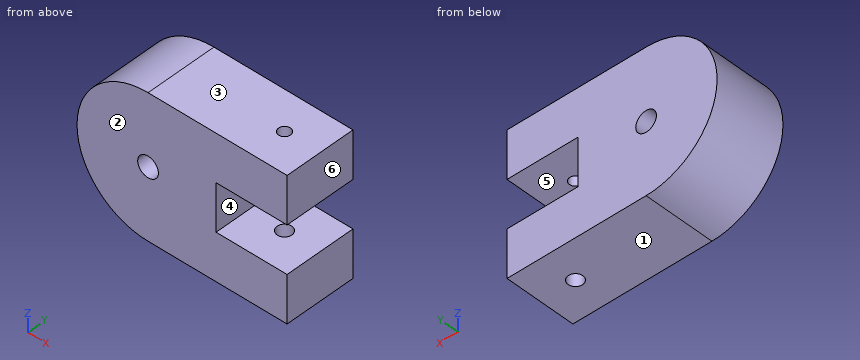
```python
from build123d import *

# Parameters (mm, degrees)
F0_R     = 11.1125
F1_DEPTH = 76.2
F3_R     = 7.9375
F4_DEPTH = 50.8
F2_R     = 6.35
F5_DEPTH = 50.8


with BuildPart() as f1:
    # F0 (on Front) → F1 (new body)
    with BuildSketch(Plane.XZ):
        with BuildLine():
            ThreePointArc((0, 152.4), (-76.2, 76.2), (0, 0))
            Line((0, 0), (149.225, 0))
            Line((149.225, 0), (149.225, 50.8))
            Line((149.225, 50.8), (73.025, 50.8))
            Line((73.025, 50.8), (73.025, 101.6))
            Line((73.025, 101.6), (149.225, 101.6))
            Line((149.225, 101.6), (149.225, 152.4))
            Line((149.225, 152.4), (0, 152.4))
        make_face()
        with Locations((0, 76.2)):
            Circle(F0_R, mode=Mode.SUBTRACT)
    extrude(amount=F1_DEPTH)

    # F3 (on face) → F4 (cut)
    with BuildSketch(Plane(origin=(0, 0, 0), x_dir=(1, 0, 0), z_dir=(0, 0, -1))):
        with Locations((111.125, 38.1)):
            Circle(F3_R)
    extrude(amount=-F4_DEPTH, mode=Mode.SUBTRACT)

    # F2 (on face) → F5 (cut)
    with BuildSketch(Plane.XY.offset(152.4)):
        with Locations((111.125, -38.1)):
            Circle(F2_R)
    extrude(amount=-F5_DEPTH, mode=Mode.SUBTRACT)


solid = f1.part
```
The listing builds one solid part. Answer for the finished solid, in the listing's coordinates (mm). Face numbers are marked on the shaded views. A direction names the side the tool comes from. Give positions to 0.01 mm unless a question says otherwise; leave off trailing zeros. Order: outer loops, then holes, each group sorted by start corner. A loop starts at its lowest first (then second) coordinate and runs counter-clockwise, first axis right, second up. Notation, with made-up numbers: (-16.5, 48.25) -> (7.5, 48.25) arc R15 cw to (7.5, 62.25) -> close; hole circle Ø8 at (17.25, 28). An arc over 180 degrees is marked (long way). Answer as CSV lines item,"result". Start each with the question number.
Q1. Given pin 1 (8 mm diameter, centred on y = -59, z = 77.5, fed in from +X) (3 decimals); pin 2 (6 mm diameter, centred on x = -28, y = -65, fed in from +Z); pin 3 (18 mm diameter, centred on x = 0, z = 76.2, fed in from -Y); pin 4 (6 mm diameter, centred on y = -21, z = 109, fed in from -X), each flat-ended and moving along its own axis, determine where each tip first touches the part or whether it passes through.
Q2. Determine the mould class of the marked faces 1, 2, 3 and 4 for opening direction Z: pulls with the +Z half, pulls with the -Z half, needs draft (parallel to the pull), parting line crosses it, or undercut.
Q3. Which of the six approach directions +Z, -Z, +X, -X, +Y, -Y give full straight-line access (tool end or side, diameter ignored) to the marked faces 5 and 6?
Q4. A cutting plane is placed at A-A (y = -38.1). Determine the outline of the cut face in (x, z) (1 decimal).
Q5. A cutting plane is placed at C-C (z = 76.2). Determine the outline of the cut face in (x, y) (1 decimal), then the cut area to 3 significant figures.
Q6. A cutting plane is placed at B-B (x = 132.5). Determine the outline of the cut face in (y, z), then the cut area to 3 significant figures.
Q7. Find the intervals of material crossed by L1, parallel to Z at x = 0, y = -49; L2, parallel to Z at x = 76, y = -26.5; L3, parallel to X at y = -47, z = 76 (3 decimals), in increasing order.
Q8. A cutting plane is placed at D-D (y = -56.5). Determine the outline of the cut face in (x, z) (1 decimal).
Results found:
1,pin 1,"x = 73.025"
1,pin 2,"z = 148.18"
1,pin 3,"through"
1,pin 4,"x = -70.13"
2,face 1,"pulls with the -Z half"
2,face 2,"needs draft"
2,face 3,"pulls with the +Z half"
2,face 4,"undercut"
3,face 5,"+X, +Y, -Y"
3,face 6,"+Z, -Z, +X, +Y, -Y"
4,outline,"(0, 0) -> (103.2, 0) -> (103.2, 50.8) -> (73, 50.8) -> (73, 101.6) -> (104.8, 101.6) -> (104.8, 152.4) -> (0, 152.4) arc R76.2 ccw to start; (117.5, 101.6) -> (149.2, 101.6) -> (149.2, 152.4) -> (117.5, 152.4) -> close; (119.1, 0) -> (149.2, 0) -> (149.2, 50.8) -> (119.1, 50.8) -> close; hole circle Ø22.2 at (0, 76.2)"
5,outline,"(-76.2, -76.2) -> (-11.1, -76.2) -> (-11.1, 0) -> (-76.2, 0) -> close; (11.1, -76.2) -> (73, -76.2) -> (73, 0) -> (11.1, 0) -> close"
5,area,"9,680 mm2"
6,outline,"(-76.2, 0) -> (0, 0) -> (0, 50.8) -> (-76.2, 50.8) -> close; (-76.2, 101.6) -> (0, 101.6) -> (0, 152.4) -> (-76.2, 152.4) -> close"
6,area,"7,740 mm2"
7,L1,"0 to 65.09, 87.31 to 152.4"
7,L2,"0 to 50.8, 101.6 to 152.4"
7,L3,"-76.2 to -11.111, 11.111 to 73.025"
8,outline,"(0, 0) -> (149.2, 0) -> (149.2, 50.8) -> (73, 50.8) -> (73, 101.6) -> (149.2, 101.6) -> (149.2, 152.4) -> (0, 152.4) arc R76.2 ccw to start; hole circle Ø22.2 at (0, 76.2)"
